Design review of the part built by this model. Coordinates are the model's own, in mm. A direction names the side the tool comes from. Give positions to 0.01 mm unless a question says otherwise; leave off trailing zeros. Order: outer loops, then holes, each group sorted by start corner. A loop starts at its lowest first (then second) coordinate and runs counter-clockwise, first axis right, second up.
```python
from build123d import *

# Parameters (mm, degrees)
SKETCH1_W          = 66
SKETCH1_H          = 48
PCB_DEPTH          = 1.6
SKETCH2_W          = 20
SKETCH2_H          = 40
HEATSINK_IN_DEPTH  = 16.4
SKETCH3_W          = 20
SKETCH3_H          = 40
HEATSINK_OUT_DEPTH = 16.4
SKETCH4_R          = 11
INDUCTOR_DEPTH     = 14.4


with BuildPart() as part:
    # Sketch1 → PCB (new body)
    with BuildSketch(Plane.XY):
        Rectangle(SKETCH1_W, SKETCH1_H)
    extrude(amount=PCB_DEPTH)

    # Sketch2 → Heatsink_in (add)
    with BuildSketch(Plane.XY.offset(1.6)):
        with Locations((-20, 0)):
            Rectangle(SKETCH2_W, SKETCH2_H)
    extrude(amount=HEATSINK_IN_DEPTH)

    # Sketch3 → Heatsink_out (add)
    with BuildSketch(Plane.XY.offset(1.6)):
        with Locations((20, 0)):
            Rectangle(SKETCH3_W, SKETCH3_H)
    extrude(amount=HEATSINK_OUT_DEPTH)

    # Sketch4 → Inductor (add)
    with BuildSketch(Plane.XY.offset(1.6)):
        Circle(SKETCH4_R)
    extrude(amount=INDUCTOR_DEPTH)


solid = part.part
```
1. Draft analysis for pull direction X (two halves, no side actions). For faces 1 (the face through (-33, 0, 1)), 2 (the face through (0, -11, 9)), 3 (the face through (20, 20, 10)), state which applies: pulls with the +X half, pulls with the -X half, needs draft (parallel to the pull), parting line crosses it, or undercut.
Recorded:
face 1: pulls with the -X half
face 2: undercut
face 3: needs draft
2. For line 1 along X through (y, z) = (-10, 2.25); line 2 along X through (y, z) = (-15.5, 12); line 3 along X through (y, z) = (7.5, 2), list the stretches that pass through material, from the lowest coordinate up.
Recorded:
line 1: x = -30 to -10, -4.58 to 4.58, 10 to 30
line 2: x = -30 to -10, 10 to 30
line 3: x = -30 to -10, -8.05 to 8.05, 10 to 30
3. Take a section at A-A (y = -12). State the section outline as (x, z) points, then the cut area to 3 significant figures.
Recorded:
outline: (-33, 0) - (33, 0) - (33, 1.6) - (30, 1.6) - (30, 18) - (10, 18) - (10, 1.6) - (-10, 1.6) - (-10, 18) - (-30, 18) - (-30, 1.6) - (-33, 1.6) - close
area: 762 mm2
4. Take a section at B-B (x = -11). State the section outline as (y, z) points, then the cut area to 3 significant figures.
Recorded:
outline: (-24, 0) - (24, 0) - (24, 1.6) - (20, 1.6) - (20, 18) - (-20, 18) - (-20, 1.6) - (-24, 1.6) - close
area: 733 mm2
5. For pin 1 (1 mm diameter, centred on y = -6, z = 5, fed in from -X); pin 2 (3 mm diameter, centred on x = 19, y = 6.5, fed in from -Z); pin 3 (4 mm diameter, centred on y = -17.5, z = 8, fed in from +X); pin 4 (6 mm diameter, centred on x = 1, z = 12.5, fed in from +Y), all flat-tipped, find the tip position at first contact; note any pin that passes through.
Recorded:
pin 1: stops at x = -30
pin 2: stops at z = 0
pin 3: stops at x = 30
pin 4: stops at y = 11
6. Take a section at C-C (z = 14). State the section outline as (x, y) points, then the cut area to 3 significant figures.
Recorded:
outline: (-30, -20) - (-10, -20) - (-10, -4.58) arc R11 ccw to (10, -4.58) - (10, -20) - (30, -20) - (30, 20) - (10, 20) - (10, 4.58) arc R11 ccw to (-10, 4.58) - (-10, 20) - (-30, 20) - close
area: 1,970 mm2
7. Machinability: for faces 4 (the face through (10, -5, 10)), 5 (the face through (-20, -20, 10)), 6 (the face through (-30, 0, 10)), 7 (the face through (-20, 20, 10)), 8 (the face through (0, 0, 16)), which of the approach directions +Z, -Z, +X, -X, +Y, -Y give a long, thin tool a straight path to every point of the face, cutting with its end or side? Answer none if there is none.
Recorded:
face 4: +Z
face 5: +Z, +X, -X, -Y
face 6: +Z, -X, +Y, -Y
face 7: +Z, +X, -X, +Y
face 8: +Z, +Y, -Y
8. Take a section at D-D (y = 8). State the section outline as (x, z) points, then the cut area to 3 significant figures.
Recorded:
outline: (-33, 0) - (33, 0) - (33, 1.6) - (30, 1.6) - (30, 18) - (10, 18) - (10, 1.6) - (7.55, 1.6) - (7.55, 16) - (-7.55, 16) - (-7.55, 1.6) - (-10, 1.6) - (-10, 18) - (-30, 18) - (-30, 1.6) - (-33, 1.6) - close
area: 979 mm2
